Part model, mm, in its own coordinate system. Face numbers are marked on the shaded views. A direction names the side the tool comes from. Round coordinates to 2 decimals unless told otherwise and drop trailing zeros. Write each loop counter-clockwise with the first axis right and the second up, starting at its lowest first coordinate (ties: lowest second). Pieces come first, ordered by that corner, then holes. Notation, with made-up numbers: (30, 32.5) -> (83, 32.5) arc R7 cw to (83, 41.5) -> close; hole circle Ø5 at (32, 78.5). An arc over 180 degrees is marked (long way). Return JSON: item names as keys, results as strings. Group by question number.
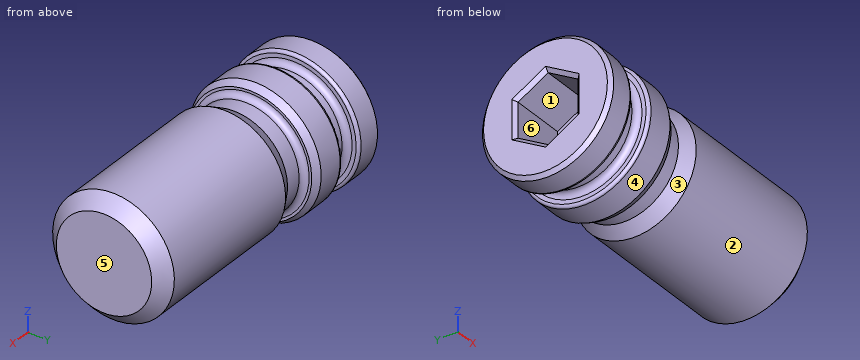
```python
from build123d import *

# Parameters (mm, degrees)
CUT_EXTRUDE1_DEPTH = 8
CHAMFER1_SIZE      = 0.5
CHAMFER2_SIZE      = 0.5
CHAMFER3_SIZE      = 1
CHAMFER3_SIZE2     = 0.577350269


with BuildPart() as part:
    # Sketch1 → Revolve1 (revolve)
    with BuildSketch(Plane.XY, mode=Mode.PRIVATE) as revolve1_sk:
        with BuildLine():
            Line((0, 0), (0, 6.525))
            Line((0, 6.525), (-1.805, 8.33))
            Line((-1.805, 8.33), (-22.929385128, 8.33))
            Line((-22.929385128, 8.33), (-24.8, 7.25))
            Line((-24.8, 7.25), (-27, 7.25))
            ThreePointArc((-27, 7.25), (-27.565685425, 7.484314575), (-27.8, 8.05))
            Line((-27.8, 8.05), (-27.8, 8.975))
            Line((-27.8, 8.975), (-32.4, 8.975))
            ThreePointArc((-32.4, 8.975), (-32.682842712, 8.857842712), (-32.8, 8.575))
            Line((-32.8, 8.575), (-32.8, 8.025))
            ThreePointArc((-32.8, 8.025), (-33.034314575, 7.459314575), (-33.6, 7.225))
            Line((-33.6, 7.225), (-35.2, 7.225))
            ThreePointArc((-35.2, 7.225), (-35.765685425, 7.459314575), (-36, 8.025))
            Line((-36, 8.025), (-36, 8.575))
            ThreePointArc((-36, 8.575), (-36.117157288, 8.857842712), (-36.4, 8.975))
            Line((-36.4, 8.975), (-40, 8.975))
            Line((-40, 8.975), (-40, 0))
            Line((-40, 0), (0, 0))
        make_face()
    revolve(revolve1_sk.sketch.rotate(Axis((0, 0, 0), (1, 0, 0)), 90), axis=Axis((0, 0, 0), (1, 0, 0)))

    # Sketch2 → Cut-Extrude1 (cut)
    with BuildSketch(Plane.ZY.offset(40)):
        Polygon((2.367136104, 4.1), (-2.367136104, 4.1), (-4.734272207, 0), (-2.367136104, -4.1), (2.367136104, -4.1), (4.734272207, 0), align=None)
    extrude(amount=-CUT_EXTRUDE1_DEPTH, mode=Mode.SUBTRACT)

    # Chamfer1
    chamfer1_edges = [part.edges().sort_by_distance(p)[0] for p in [
        (-40, 2.05, 3.550704156),
        (-40, 4.1, 0),
        (-40, 2.05, -3.550704156),
        (-40, -2.05, -3.550704156),
        (-40, -4.1, 0),
        (-40, -2.05, 3.550704156),
    ]]
    chamfer(chamfer1_edges, length=CHAMFER1_SIZE)

    # Chamfer2
    chamfer2_edges = [part.edges().sort_by_distance(p)[0] for p in [
        (-40, 0, -8.975),
    ]]
    chamfer(chamfer2_edges, length=CHAMFER2_SIZE)

    # Chamfer3
    chamfer3_edges = [part.edges().sort_by_distance(p)[0] for p in [
        (-27.8, 0, -8.975),
    ]]
    chamfer3_side = [part.faces().sort_by_distance(p)[0] for p in [
        (-30.1, 0, -8.975),
    ]]
    chamfer(chamfer3_edges, length=CHAMFER3_SIZE, length2=CHAMFER3_SIZE2, reference=chamfer3_side[0])


solid = part.part
```
Item 1: Wall check: L1, parallel to X at y = -2.25, z = -7; L2, parallel to X at y = 3, z = -7; L3, parallel to X at y = 0.75, z = 4. Give the ranges that are in metal, low to high.
Item 2: Flat gauge pins, fed straight in: P1, Ø1, axis at x = -27, y = -6.5, coming from the -Z side; P2, Ø1.5, axis at y = -2, z = 0.5, coming from the -X side; P3, Ø4, axis at x = -10.5, y = 4.5, coming from the +Z side. Where does each tip first touch, or does it go through?
Item 3: Two-plate mould, pull along Y, no slides. Class the marked faces 4, 5 and 6: released by +Y, released by -Y, zero draft, split by the parting line, or undercut.
Item 4: Cut at B-B (x = -11.5). Write the cut outline in (y, z), then the cut area to 3 significant figures.
Item 5: Cut at A-A (x = -37). Write the cut outline in (y, z) (3 decimals), then the cut area to 3 significant figures.
Item 6: Which spindle directions (+Z, -Z, +X, -X, +Y, -Y) get a long thin tool onto all of the face, cutting with end or side? Do the marked faces 1, 2 and 3. Say none if no direction does.
Checks:
{
 "1": {"L1": "x = -40 to -35.63, -33.17 to -27.39, -24.62 to -0.83", "L2": "x = -40 to -35.89, -32.91 to -27.67, -24.17 to -1.09", "L3": "x = -32 to 0"},
 "2": {"P1": "stops at z = -4.07", "P2": "stops at x = -32", "P3": "stops at z = 7.95"},
 "3": {"face 4": "split by the parting line", "face 5": "zero draft", "face 6": "undercut"},
 "4": {"outline": "circle Ø16.66 at (0, 0)", "area": "218 mm2"},
 "5": {"outline": "circle Ø17.95 at (0, 0); hole (-4.1, -2.367) -> (0, -4.734) -> (4.1, -2.367) -> (4.1, 2.367) -> (0, 4.734) -> (-4.1, 2.367) -> close", "area": "195 mm2"},
 "6": {"face 1": "-X", "face 2": "+X", "face 3": "none"}
}
